For this review, take the finished solid that the model builds, in its own axes (mm). A direction names the side the tool comes from. Round coordinates to 2 decimals unless told otherwise and drop trailing zeros. Loops run counter-clockwise (first coordinate to the right, second up) from the corner with the lowest first, then second, coordinate; pieces in that order, holes last.
1. Consider section B-B on y = 9.5. State the section outline as (x, z) points.
2. To check wall thickness, follow line 1 along X through (y, z) = (3.75, 16); line 2 along Z through (x, y) = (17, 6); line 3 along Y through (x, z) = (17.65, 45.5). State the ranges of each line that lie inside material, in increasing order.
3. Consider section A-A on z = 5. State the section outline as (x, y) points.
4. Consider section D-D on z = 21. State the section outline as (x, y) points, then the cut area to 3 significant figures.
5. Consider section C-C on x = 14.5. State the section outline as (y, z) points.
6. Tool access review of faces 4 (the flat face through (17, 8.5, 44)), 5 (the flat face through (18.5, 6, 43.6)), 6 (the flat face through (16, 2, 25)), 7 (the flat face through (17, 3.5, 44)), 8 (the flat face through (16, 1, 20)): name each direction out of +Z, -Z, +X, -X, +Y, -Y from which nothing blocks a thin tool from reaching the whole face with its end or side.
7. Draft analysis for pull direction Z (two halves, no side actions). For faces 1 (the cylindrical face through (17.232, 6.421, 46.835)), 2 (the flat face through (0, 6, 21)), 3 (the flat face through (16, 7, 40)), state which applies: released by +Z, released by -Z, zero draft, split by the parting line, or undercut.
8. Clearance check with flat-ended pins moving along their axes: pin 1 Ø1 at (x, y) = (18, 10) entering from +Z; pin 2 Ø1.5 at (x, y) = (10.5, 5) entering from -Z; pin 3 Ø1 at (x, y) = (17, 1) entering from -Z. State where each tip first meets the part, or that it passes through.
Autodesk Inventor part; units mm, degrees
ref_plane "YZ Plane" through (0, 0, 0) normal (1, 0, 0) x (0, 1, 0)
ref_plane "XZ Plane" through (0, 0, 0) normal (0, 1, 0) x (-1, 0, 0)
ref_plane "XY Plane" through (0, 0, 0) normal (0, 0, 1) x (1, 0, 0)
sketch "Sketch1" plane through (0, 0, 0) normal (0, 1, 0) x (-1, 0, 0)
  line L0 (0, 0) -> (-32, 0)
  line L1 (-32, 0) -> (-32, 42)
  line L2 (-32, 42) -> (0, 42)
  line L3 (0, 42) -> (0, 0)
  dimension "d0" = 32
  dimension "d1" = 42
extrude "Extrusion1" add sketch "Sketch1" along normal blind 2
sketch "Sketch2" plane through (0, 2, 0) normal (0, 1, 0) x (1, 0, 0)
  line L0 (0, -42) -> (32, -42)
  line L1 (0, 0) -> (32, 0)
  line L2 (32, 0) -> (32, -42)
  line L3 (32, -42) -> (0, -42)
  line L4 (0, -42) -> (0, 0)
  line L5 (0, 0) -> (0, -42)
  line L6 (0, 0) -> (2, 0)
  line L7 (2, 0) -> (2, -2)
  line L8 (2, -2) -> (0, -2)
  line L9 (0, -2) -> (0, 0)
  line L10 (32, -42) -> (30, -42)
  line L11 (30, -42) -> (30, -40)
  line L12 (30, -40) -> (32, -40)
  line L13 (32, -40) -> (32, -42)
  line L14 (30, -40) -> (2, -40)
  line L15 (2, -40) -> (2, -2)
  line L16 (2, -2) -> (30, -2)
  line L17 (30, -2) -> (30, -40)
  line L18 (32, -42) -> (32, 0)
  line L19 (30, -2) -> (32, -2)
  line L20 (32, -2) -> (32, 0)
  line L21 (32, 0) -> (30, 0)
  line L22 (30, 0) -> (30, -2)
  dimension "d4" = 2
  dimension "d5" = 2
  dimension "d6" = 2
  dimension "d7" = 2
extrude "Extrusion2" add sketch "Sketch2" along normal blind 10 contours L4 L8 L15 L14 L11 L0 | L11 L12 L2 L0 | L4 L1 L7 L8 | L17 L19 L2 L12 | L22 L1 L2 L19
sketch "Sketch3" plane through (0, 2, 0) normal (0, 1, 0) x (1, 0, 0)
  line L0 (30, 0) -> (2, 0)
  line L1 (30, 0) -> (30, -40)
  line L2 (2, 0) -> (30, 0)
  line L3 (30, 0) -> (30, -40)
  line L4 (30, -40) -> (2, -40)
  line L5 (2, -40) -> (2, 0)
  line L6 (2, 0) -> (6, 0)
  line L7 (6, 0) -> (6, -4)
  line L8 (6, -4) -> (2, -4)
  line L9 (2, -4) -> (2, 0)
  line L10 (30, 0) -> (26, 0)
  line L11 (26, 0) -> (26, -4)
  line L12 (26, -4) -> (30, -4)
  line L13 (30, -4) -> (30, 0)
  line L14 (6, 0) -> (26, 0)
  line L15 (26, 0) -> (26, -20)
  line L16 (26, -20) -> (6, -20)
  line L17 (6, -20) -> (6, 0)
  point P0 (0, 0)
  dimension "d10" = 4
  dimension "d11" = 4
  dimension "d12" = 4
  dimension "d13" = 4
  dimension "d14" = 20
  dimension "d15" = 20
extrude "Extrusion3" cut sketch "Sketch3" against normal through all contours L11 L15 L16 L17 L7 L0
sketch "Sketch4" plane through (0, 0, 42) normal (0, 0, 1) x (1, 0, 0)
  line L0 (2, 12) -> (0, 12)
  line L1 (32, 0) -> (26, 0)
  line L2 (0, 12) -> (32, 12)
  line L3 (32, 12) -> (32, 0)
  line L4 (32, 0) -> (0, 0)
  line L5 (0, 0) -> (0, 12)
  line L6 (0, 12) -> (13.5, 12)
  line L7 (13.5, 12) -> (13.5, 8.5)
  line L8 (13.5, 8.5) -> (0, 8.5)
  line L9 (0, 8.5) -> (0, 12)
  line L10 (13.5, 8.5) -> (18.5, 8.5)
  line L11 (18.5, 8.5) -> (18.5, 3.5)
  line L12 (18.5, 3.5) -> (13.5, 3.5)
  line L13 (13.5, 3.5) -> (13.5, 8.5)
  line L14 (18.5, 8.5) -> (16, 8.5)
  line L15 (16, 8.5) -> (16, 3.5)
  line L16 (16, 3.5) -> (18.5, 3.5)
  line L17 (18.5, 3.5) -> (18.5, 8.5)
  dimension "d18" = 13.5
  dimension "d19" = 3.5
  dimension "d20" = 5
  dimension "d21" = 5
extrude "Extrusion4" add sketch "Sketch4" along normal blind 6 contours L10 L11 L12 L15
sketch "Sketch5" plane through (16, 3.5, 42) normal (-1, 0, 0) x (0, 0, 1)
  line L0 (6, 0) -> (6, 5)
  line L1 (6, 5) -> (3.5, 5)
  line L2 (3.5, 5) -> (3.5, 2.5)
  line L3 (3.5, 2.5) -> (6, 2.5)
  line L4 (6, 2.5) -> (6, 5)
  circle A0 centre (3.5, 2.5) radius 1.4
  point P0 (-42, -3.5)
  dimension "d24" = 2.5
  dimension "d25" = 2.5
  dimension "d26" = 2.8
extrude "Extrusion5" cut sketch "Sketch5" against normal through all contours A0 L2 L3 | L3 L2 A0
fillet "Fillet1" radius 2.5 2 edges at (17.25, 8.5, 48) (17.25, 3.5, 48)
properties part number "CAM04"
Resolved:
1. outline: (0, 0) - (2, 0) - (2, 40) - (30, 40) - (30, 0) - (32, 0) - (32, 42) - (0, 42) - close
2. line 1: x = 0 to 2, 30 to 32
2. line 2: z = 40 to 44.1, 46.9 to 48
2. line 3: y = 3.5 to 4.6, 7.4 to 8.5
3. outline: (0, 0) - (6, 0) - (6, 2) - (2, 2) - (2, 12) - (0, 12) - close; (26, 0) - (32, 0) - (32, 12) - (30, 12) - (30, 2) - (26, 2) - close
4. outline: (0, 0) - (32, 0) - (32, 12) - (30, 12) - (30, 2) - (2, 2) - (2, 12) - (0, 12) - close
4. area: 104 mm2
5. outline: (0, 20) - (2, 20) - (2, 40) - (12, 40) - (12, 42) - (0, 42) - close
6. face 4: +Z, +X, -X, +Y
6. face 5: +Z, +X, +Y, -Y
6. face 6: -Z, +Y
6. face 7: +Z, +X, -X, -Y
6. face 8: -Z, +Y, -Y
7. face 1: undercut
7. face 2: zero draft
7. face 3: released by -Z
8. pin 1: stops at z = 42
8. pin 2: stops at z = 40
8. pin 3: stops at z = 20
